The listing builds one solid part. Answer for the finished solid, in the listing's coordinates (mm). Face numbers are marked on the shaded views. A direction names the side the tool comes from. Give positions to 0.01 mm unless a question says otherwise; leave off trailing zeros. Write each loop counter-clockwise with the first axis right and the second up, starting at its lowest first coordinate (ties: lowest second). Pieces come first, ordered by that corner, then holes. Notation, with made-up numbers: (44.5, 75.5) - (76.5, 75.5) arc R17 cw to (76.5, 101.5) - close; hole circle Ø2 at (54, 44). An arc over 180 degrees is marked (long way). One line per question, with ' | ' between items. Start each with the question number.
1. Given P1, Ø2.5, axis at x = 4, z = -27, coming from the -Y side; P2, Ø8, axis at y = -4.5, z = 36, coming from the -X side; P3, Ø2, axis at y = -8, z = 3, coming from the +X side; P4, Ø3.5, axis at x = -7.5, y = -7.5, coming from the -Z side, each flat-ended and moving along its own axis, determine where each tip first touches the part or whether it passes through.
2. For the marked faces 4, 5 and 6, determine the directions among +Z, -Z, +X, -X, +Y, -Y from which every point of the face is accessible in a straight line to the end or side of a thin tool.
3. Find the intervals of material crossed by L1, parallel to X at y = -5.5, z = 9; L2, parallel to Z at x = -1.5, y = 1; L3, parallel to Z at x = -4, y = 2.25, in increasing order. Write a range as from..to.
4. The mould has two halves that part along Z. Classify the marked faces 1, 2 and 3: +Z half, -Z half, draft (parallel to the pull), parting line (faces both ways), or undercut.
5. A cutting plane is placed at A-A (z = -9). Determine the outline of the cut face in (x, y).
6. A cutting plane is placed at D-D (z = -26). Determine the outline of the cut face in (x, y).
7. A cutting plane is placed at B-B (x = 0). State how many separate pieces and enclosed holes the cut face has, then the cut area to 3 significant figures.
```python
from build123d import *

# Parameters (mm, degrees)
SKETCH1_R           = 2.25
BOSS_EXTRUDE1_DEPTH = 12
FILLET1_R           = 5
CUT_EXTRUDE1_START  = 50
SKETCH2_R           = 2.25
CUT_EXTRUDE1_DEPTH  = 5
FILLET3_R           = 2
FILLET2_R           = 5
CHAMFER1_SIZE       = 1


with BuildPart() as part:
    # Sketch1 → Boss-Extrude1 (new body, symmetric)
    with BuildSketch(Plane(origin=(0, 0, 0), x_dir=(1, 0, 0), z_dir=(0, 1, 0))):
        Polygon((8, 0), (4, 0), (0, -8), (0, -10), (4, -18), (0, -26), (0, -28), (4, -36), (0, -44), (0, -50), (12, -50), (8, -27.314872722), align=None)
        with Locations((4, -27)):
            Circle(SKETCH1_R, mode=Mode.SUBTRACT)
        with Locations((4, -9)):
            Circle(SKETCH1_R, mode=Mode.SUBTRACT)
    extrude(amount=BOSS_EXTRUDE1_DEPTH, both=True)

    # Fillet1
    fillet1_edges = [part.edges().sort_by_distance(p)[0] for p in [
        (4, 0, 18),
        (4, 0, 36),
    ]]
    fillet(fillet1_edges, radius=FILLET1_R)

    # Mirror1: part across plane


with BuildPart() as part_1:
    add(part.part)
    add(part.part.mirror(Plane(origin=(0, 0, 0), x_dir=(0, 0, 1), z_dir=(1, 0, 0))))

    # Sketch2 → Cut-Extrude1 (cut)
    with BuildSketch(Plane.XY.offset(CUT_EXTRUDE1_START)):
        with Locations((-7.5, 7.5)):
            Circle(SKETCH2_R)
        Circle(SKETCH2_R)
        with Locations((7.5, 7.5)):
            Circle(SKETCH2_R)
        with Locations((7.5, -7.5)):
            Circle(SKETCH2_R)
        with Locations((-7.5, -7.5)):
            Circle(SKETCH2_R)
    extrude(amount=-CUT_EXTRUDE1_DEPTH, mode=Mode.SUBTRACT)

    # Fillet3
    fillet3_edges = [part_1.edges().sort_by_distance(p)[0] for p in [
        (0, 0, 44),
        (0, 0, 8),
        (0, 0, 10),
        (0, 0, 26),
        (0, 0, 28),
    ]]
    fillet(fillet3_edges, radius=FILLET3_R)

    # Mirror2: part across plane


with BuildPart() as part_2:
    add(part_1.part)
    add(part_1.part.mirror(Plane.XY))

    # Fillet2
    fillet2_edges = [part_2.edges().sort_by_distance(p)[0] for p in [
        (4, 0, 0),
        (-4, 0, 0),
    ]]
    fillet(fillet2_edges, radius=FILLET2_R)

    # Chamfer1
    chamfer1_edges = [part_2.edges().sort_by_distance(p)[0] for p in [
        (2.335410197, -12, 32.670820393),
        (2.335410197, 12, 32.670820393),
        (-2.335410197, -12, 32.670820393),
        (-2.335410197, 12, 32.670820393),
        (2.335410197, -12, 14.670820393),
        (2.335410197, 12, 14.670820393),
        (-2.335410197, -12, 14.670820393),
        (-2.335410197, 12, 14.670820393),
        (0, -12, 30.472135955),
        (0, 12, 30.472135955),
        (0, -12, 12.472135955),
        (0, 12, 12.472135955),
        (0, -12, 5.527864045),
        (0, 12, 5.527864045),
        (0, -12, 23.527864045),
        (0, 12, 23.527864045),
        (0, -12, 41.527864045),
        (0, 12, 41.527864045),
        (2.335410197, 12, -32.670820393),
        (2.335410197, 12, -39.329179607),
        (10, -12, -38.657436361),
        (2.335410197, 12, -14.670820393),
        (2.335410197, 12, -21.329179607),
        (-2.335410197, 12, -32.670820393),
        (-3.409830056, 12, -36),
        (-2.335410197, 12, -39.329179607),
        (10, 12, -38.657436361),
        (-2.335410197, 12, -14.670820393),
        (-3.409830056, 12, -18),
        (-2.335410197, 12, -21.329179607),
        (-3.409830056, -12, -36),
        (2.335410197, -12, -32.670820393),
        (2.335410197, -12, -39.329179607),
        (-10, -12, -38.657436361),
        (2.335410197, -12, -14.670820393),
        (2.335410197, -12, -21.329179607),
        (-3.409830056, -12, -18),
        (3.409830056, 12, -18),
        (3.409830056, -12, -18),
        (3.409830056, 12, -36),
        (3.409830056, -12, -36),
        (-2.335410197, -12, -32.670820393),
        (-2.335410197, -12, -39.329179607),
        (-10, 12, -38.657436361),
        (-2.335410197, -12, -14.670820393),
        (-2.335410197, -12, -21.329179607),
        (0, 12, -30.472135955),
        (0, -12, -30.472135955),
        (0, 12, -12.472135955),
        (0, -12, -12.472135955),
        (0, 12, -5.527864045),
        (0, -12, -5.527864045),
        (0, 12, -23.527864045),
        (0, -12, -23.527864045),
        (0, 12, -41.527864045),
        (0, -12, -41.527864045),
        (8, -12, 0),
        (10, -12, 38.657436361),
        (-2.335410197, 12, -3.329179607),
        (-2.335410197, -12, -3.329179607),
        (-2.335410197, 12, 3.329179607),
        (-2.335410197, -12, 3.329179607),
        (2.335410197, -12, 3.329179607),
        (2.335410197, 12, 3.329179607),
        (2.335410197, -12, -3.329179607),
        (2.335410197, 12, -3.329179607),
        (-3.409830056, -12, 0),
        (-3.409830056, 12, 0),
        (3.409830056, -12, 0),
        (3.409830056, 12, 0),
        (10, 12, 38.657436361),
        (8, 12, 0),
        (2.335410197, -12, 21.329179607),
        (2.335410197, 12, 21.329179607),
        (2.335410197, -12, 39.329179607),
        (2.335410197, 12, 39.329179607),
        (3.409830056, -12, 18),
        (3.409830056, 12, 18),
        (3.409830056, -12, 36),
        (3.409830056, 12, 36),
        (-2.335410197, 12, 39.329179607),
        (-10, -12, 38.657436361),
        (-8, -12, 0),
        (-2.335410197, 12, 21.329179607),
        (-8, 12, 0),
        (-10, 12, 38.657436361),
        (-2.335410197, -12, 39.329179607),
        (-2.335410197, -12, 21.329179607),
        (-3.409830056, 12, 18),
        (-3.409830056, -12, 18),
        (-3.409830056, 12, 36),
        (-3.409830056, -12, 36),
    ]]
    chamfer(chamfer1_edges, length=CHAMFER1_SIZE)


solid = part_2.part
```
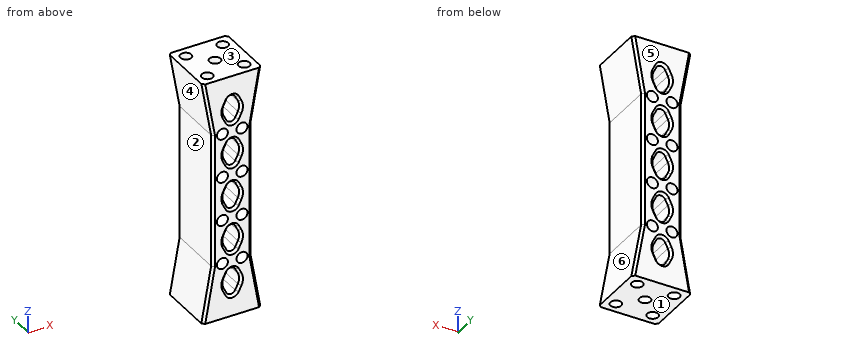
Determined:
1) P1: through | P2: x = -10.24 | P3: x = 8 | P4: z = -45
2) face 4: -X, +Y, -Y | face 5: +Z, -Z, +X, -X, +Y | face 6: +X, +Y, -Y
3) L1: -8..-6.25, -1.75..1.75, 6.25..8 | L2: -45..-40.85, -31.15..-22.85, -13.15..-4.85, 4.85..13.15, 22.85..31.15, 40.85..45 | L3: -50..-29.25, -24.75..-11.25, -6.75..6.75, 11.25..24.75, 29.25..50
4) face 1: -Z half | face 2: undercut | face 3: +Z half
5) outline: (-8, -11) - (-7, -12) - (-6.25, -12) - (-6.25, 12) - (-7, 12) - (-8, 11) - close; (-1.75, -12) - (1.75, -12) - (1.75, 12) - (-1.75, 12) - close; (6.25, -12) - (7, -12) - (8, -11) - (8, 11) - (7, 12) - (6.25, 12) - close
6) outline: (-8, -11) - (-7, -12) - (-6.02, -12) - (-6.02, 12) - (-7, 12) - (-8, 11) - close; (-1.98, -12) - (1.98, -12) - (1.98, 12) - (-1.98, 12) - close; (6.02, -12) - (7, -12) - (8, -11) - (8, 11) - (7, 12) - (6.02, 12) - close
7) separate pieces: 6 | enclosed holes: 0 | area: 1,020 mm2
